from build123d import *

# Parameters (mm, degrees)
SKETCH_1_W          = 13
SKETCH_1_H          = 30
EXTRUDE_1_DEPTH     = 10
SKETCH_2_W          = 6
SKETCH_2_H          = 28
CUT_EXTRUDE_1_DEPTH = 10
SKETCH_3_R          = 1.5
CUT_EXTRUDE_2_DEPTH = 58.605092201
SKETCH_4_R          = 1.5
CUT_EXTRUDE_3_DEPTH = 58.605092201


with BuildPart() as part:
    # 草图1 → 凸台-拉伸1 (new body)
    with BuildSketch(Plane.XY):
        Rectangle(SKETCH_1_W, SKETCH_1_H)
        Polygon((16.481333294, -54.283628291), (15.495607284, -15), (6.5, -15), (-6.5, -15), (-6.5, -35), align=None)
    extrude(amount=EXTRUDE_1_DEPTH)

    # 草图2 → 切除-拉伸1 (cut)
    with BuildSketch(Plane(origin=(6.5, 0, 0), x_dir=(0, 0, -1), z_dir=(1, 0, 0))):
        with Locations((-5, 1)):
            Rectangle(SKETCH_2_W, SKETCH_2_H)
    extrude(amount=-CUT_EXTRUDE_1_DEPTH, mode=Mode.SUBTRACT)

    # 草图3 → 切除-拉伸2 (cut, through all)
    with BuildSketch(Plane.XY.offset(10)):
        with Locations((1.5, 12)):
            Circle(SKETCH_3_R)
    extrude(amount=-CUT_EXTRUDE_2_DEPTH, mode=Mode.SUBTRACT)

    # 草图4 → 切除-拉伸3 (cut, through all)
    with BuildSketch(Plane.XY.offset(10)):
        with Locations((1.5, -8)):
            Circle(SKETCH_4_R)
    extrude(amount=-CUT_EXTRUDE_3_DEPTH, mode=Mode.SUBTRACT)


solid = part.part
Read the model definition and answer for the solid it produces. Units are mm, in the model's axes. A direction names the side the tool comes from. Round coordinates to 2 decimals unless told otherwise and drop trailing zeros. Write each loop counter-clockwise with the first axis right and the second up, starting at its lowest first coordinate (ties: lowest second). Pieces come first, ordered by that corner, then holes. Notation, with made-up numbers: (51, 85) - (101, 85) arc R25 ccw to (101, 113) - close; hole circle Ø8 at (-38, -4.5). An arc over 180 degrees is marked (long way). Use a Markdown table: item, result.
(1) Straight lines are drawn through the part: line 1 along Z through (x, y) = (-3, 4); line 2 along Y through (x, z) = (1.5, 8.8); line 3 along X through (y, z) = (11, 3.25). For each, find the intervals that lie inside material, in ascending order. Write a range as [from, to].
Reported:
| item | result |
|---|---|
| line 1 | [0, 2], [8, 10] |
| line 2 | [-41.71, -9.5], [-6.5, 10.5], [13.5, 15] |
| line 3 | [-6.5, -3.5] |
(2) The part is cut by section D-D (z = 1.25). Write down the section's boundary in (x, y).
Reported:
| item | result |
|---|---|
| outline | (-6.5, -35) - (16.48, -54.28) - (15.5, -15) - (6.5, -15) - (6.5, 15) - (-6.5, 15) - close; hole circle Ø3 at (1.5, -8); hole circle Ø3 at (1.5, 12) |
(3) The mould has two halves that part along X. Classify faces 4 (the flat face through (2, -13, 5)), 5 (the flat face through (4.83, -44.507, 4.93)), 6 (the cylindrical face through (0.3, 11.1, 9)), 7 (the cylindrical face through (1.175, -9.464, 9.014)): released by +X, released by -X, zero draft, split by the parting line, or undercut.
Reported:
| item | result |
|---|---|
| face 4 | zero draft |
| face 5 | released by -X |
| face 6 | undercut |
| face 7 | undercut |
(4) Each of these flat-tipped pins is pushed along its axis until it touches: pin 1 Ø3 at (y, z) = (5.5, 7) entering from +X; pin 2 Ø3 at (y, z) = (-28.5, 6.5) entering from +X; pin 3 Ø2 at (x, z) = (9, 9) entering from -Y. Where does it stop, or does it pass through?
Reported:
| item | result |
|---|---|
| pin 1 | x = 6.5 |
| pin 2 | x = 15.87 |
| pin 3 | y = -48.85 |
(5) The part is cut by section C-C (y = -8). Write down the section's boundary in (x, z), then the cut area to 3 significant figures.
Reported:
| item | result |
|---|---|
| outline | (-6.5, 0) - (0, 0) - (0, 2) - (-3.5, 2) - (-3.5, 8) - (0, 8) - (0, 10) - (-6.5, 10) - close; (3, 0) - (6.5, 0) - (6.5, 2) - (3, 2) - close; (3, 8) - (6.5, 8) - (6.5, 10) - (3, 10) - close |
| area | 58.0 mm2 |
(6) Which of the six approach directions +Z, -Z, +X, -X, +Y, -Y give full straight-line access (tool end or side, diameter ignored) to faces 1 (the flat face through (5, -19, 0)), 2 (the flat face through (2, 1, 2)), 3 (the flat face through (6.5, -0.2, 1.6))?
Reported:
| item | result |
|---|---|
| face 1 | -Z, +X, -X, +Y, -Y |
| face 2 | +X, +Y |
| face 3 | +Z, -Z, +X, +Y |
(7) The part is cut by section B-B (y = 6.5). Write down the section's boundary in (x, z), then the cut area to 3 significant figures.
Reported:
| item | result |
|---|---|
| outline | (-6.5, 0) - (6.5, 0) - (6.5, 2) - (-3.5, 2) - (-3.5, 8) - (6.5, 8) - (6.5, 10) - (-6.5, 10) - close |
| area | 70.0 mm2 |
(8) The part is cut by section A-A (z = 6.75). Write down the section's boundary in (x, y), then the cut area to 3 significant figures.
Reported:
| item | result |
|---|---|
| outline | (-6.5, -35) - (16.48, -54.28) - (15.5, -15) - (6.5, -15) - (6.5, -13) - (-3.5, -13) - (-3.5, 15) - (-6.5, 15) - close |
| area | 772 mm2 |
